Autodesk Inventor part; units mm, degrees
ref_plane "YZ Plane" through (0, 0, 0) normal (1, 0, 0) x (0, 1, 0)
ref_plane "XZ Plane" through (0, 0, 0) normal (0, 1, 0) x (-1, 0, 0)
ref_plane "XY Plane" through (0, 0, 0) normal (0, 0, 1) x (1, 0, 0)
sketch "Sketch1" plane through (0, 0, 0) normal (0, 1, 0) x (-1, 0, 0)
  line L0 (0, 0) -> (254, 0)
  line L1 (254, 0) -> (254, -127)
  line L2 (254, -127) -> (0, -127)
  line L3 (0, -127) -> (0, 0)
  circle A0 centre (17.9672, -8.2233) radius 1.905
  circle A1 centre (17.9672, -48.8633) radius 1.905
  circle A2 centre (58.6072, -48.8633) radius 1.905
  circle A3 centre (58.6072, -8.2233) radius 1.905
  circle A4 centre (67.644, -79.6665) radius 1.905
  circle A5 centre (67.644, -108.6225) radius 1.905
  circle A6 centre (8.462, -79.6665) radius 1.905
  circle A7 centre (8.462, -108.6225) radius 1.905
  circle A8 centre (236.9221, -63.5) radius 3.81
  circle A9 centre (167.3261, -63.5) radius 3.175
  circle A10 centre (150.3735, -19.2274) radius 1.905
  circle A11 centre (150.3735, -108.8774) radius 1.905
  circle A12 centre (88.1435, -108.8774) radius 1.905
  circle A13 centre (88.1435, -19.2274) radius 1.905
  circle A14 centre (204.3299, -47.9) radius 1.905
  circle A15 centre (204.3299, -77.11) radius 1.905
  circle A16 centre (185.7625, -77.11) radius 1.905
  circle A17 centre (185.7625, -47.9) radius 1.905
  dimension "d0" = 254
  dimension "d1" = 127
  dimension "d2" = 3.81
  dimension "d3" = 3.81
  dimension "d4" = 3.81
  dimension "d5" = 3.81
  dimension "d6" = 40.64
  dimension "d7" = 40.64
  dimension "d8" = 40.64
  dimension "d9" = 40.64
  dimension "d14" = 3.81
  dimension "d15" = 3.81
  dimension "d16" = 3.81
  dimension "d17" = 3.81
  dimension "d18" = 7.62
  dimension "d19" = 63.5
  dimension "d20" = 6.35
  dimension "d21" = 69.596
  dimension "d22" = 63.5
  dimension "d25" = 3.81
  dimension "d26" = 3.81
  dimension "d27" = 3.81
  dimension "d28" = 3.81
  dimension "d31" = 3.81
  dimension "d32" = 3.81
  dimension "d33" = 3.81
  dimension "d34" = 3.81
extrude "Extrusion1" add sketch "Sketch1" along normal blind 6.35
properties part number "BaseBoard"
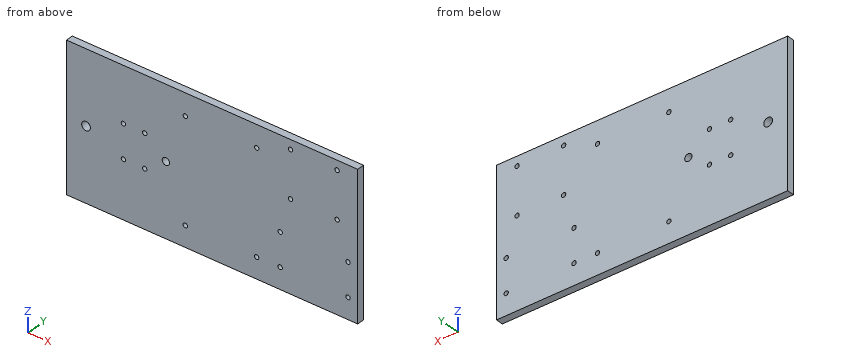
Work out the finished part from the listing and answer in its coordinate system (mm). Coordinates: 2 decimals unless noted, no trailing zeros. Loops run counter-clockwise (first coordinate to the right, second up) from the corner with the lowest first, then second, coordinate; pieces in that order, holes last. Notation, with made-up numbers: M 38.25,-28 L 81.25,-28 A13 ccw 81.25,-17 Z; hole C 80.25,31 d2. An arc over 180 degrees is marked long. Use CSV: the item, a comma, the result in double quotes. Start each with the question number.
(1) Consider line 1 (Z direction, x = -67.5, y = 3); line 2 (X direction, y = 2, z = -77.11); line 3 (X direction, y = 3, z = -62.5). Determine where each line is inside the solid, lowest interval first.
(2) Given pin 1 Ø6 at (x, z) = (-67.64, -79.67) entering from +Y, flat-ended and moving along its own axis, determine where the tip first touches the part or whether it passes through.
(3) Find section A-A, the plane z = -63.5. Give the vertices of the cut face in (x, y), then the cut area to 3 significant figures.
Recorded:
1,line 1,"z = -127 to -110.52, -106.72 to -81.57, -77.77 to 0"
1,line 2,"x = -254 to -206.23, -202.42 to -187.67, -183.86 to 0"
1,line 3,"x = -254 to -240.6, -233.25 to -170.34, -164.31 to 0"
2,pin 1,"stops at y = 6.35"
3,outline,"M -254,0 L -240.73,0 L -240.73,6.35 L -254,6.35 Z; M -233.11,0 L -170.5,0 L -170.5,6.35 L -233.11,6.35 Z; M -164.15,0 L 0,0 L 0,6.35 L -164.15,6.35 Z"
3,area,"1,520 mm^2"
